Read the model definition and answer for the solid it produces. Units are mm, in the model's axes. A direction names the side the tool comes from. Coordinates: 2 decimals unless noted, no trailing zeros. Write each loop counter-clockwise with the first axis right and the second up, starting at its lowest first coordinate (ties: lowest second). Pieces come first, ordered by that corner, then holes. Notation, with made-up numbers: (-10, 61) - (16, 61) arc R18 cw to (16, 79) - close; hole circle Ø11 at (79.25, -39.5). An arc over 180 degrees is marked (long way). Return JSON: item names as keys, results as strings.
```python
from build123d import *

# Parameters (mm, degrees)
SKETCH1_W           = 69
SKETCH1_H           = 40
BOSS_EXTRUDE1_DEPTH = 5.08
SKETCH2_W           = 23
SKETCH2_H           = 5.08
BOSS_EXTRUDE2_DEPTH = 5.08
CUT_EXTRUDE4_DEPTH  = 5.08


with BuildPart() as part:
    # Sketch1 → Boss-Extrude1 (new body)
    with BuildSketch(Plane(origin=(0, 0, 0), x_dir=(1, 0, 0), z_dir=(0, 1, 0))):
        with Locations((-34.5, 20)):
            Rectangle(SKETCH1_W, SKETCH1_H)
    extrude(amount=BOSS_EXTRUDE1_DEPTH)

    # Sketch2 → Boss-Extrude2 (add)
    with BuildSketch(Plane.XY):
        with Locations((-57.5, 2.54)):
            Rectangle(SKETCH2_W, SKETCH2_H)
        with Locations((-11.5, 2.54)):
            Rectangle(SKETCH2_W, SKETCH2_H)
    extrude(amount=BOSS_EXTRUDE2_DEPTH)

    # Sketch7 → Cut-Extrude4 (cut)
    with BuildSketch(Plane(origin=(0, 5.08, 0), x_dir=(1, 0, 0), z_dir=(0, 1, 0))):
        with BuildLine():
            ThreePointArc((-28.25, 10), (-34.5, 16.25), (-40.75, 10))
            Line((-40.75, 10), (-28.25, 10))
        make_face()
        with BuildLine():
            Line((-28.25, 10), (-40.75, 10))
            ThreePointArc((-40.75, 10), (-34.5, 3.75), (-28.25, 10))
        make_face()
        with BuildLine():
            Line((-40.75, 40), (-40.75, 10))
            ThreePointArc((-40.75, 10), (-34.5, 16.25), (-28.25, 10))
            Line((-28.25, 10), (-28.25, 40))
            Line((-28.25, 40), (-40.75, 40))
        make_face()
    extrude(amount=-CUT_EXTRUDE4_DEPTH, mode=Mode.SUBTRACT)


solid = part.part
```
(1) Which of the six approach directions +Z, -Z, +X, -X, +Y, -Y give full straight-line access (tool end or side, diameter ignored) to faces 4 (the face through (-28.25, 3, -25)), 5 (the face through (-43, 5.08, -18)), 6 (the face through (-46, 3, 3))?
Answer:
{"face 4": "-Z, +Y, -Y", "face 5": "+Z, -Z, +X, -X, +Y", "face 6": "+Z, +Y, -Y"}
(2) Determine the mould class of faces 1 (the face through (-40.75, 3, -25)), 2 (the face through (0, 3, -17)), 3 (the face through (-55, 3, -40)) for opening direction X: +X half, -X half, draft (parallel to the pull), parting line (faces both ways), or undercut.
Answer:
{"face 1": "undercut", "face 2": "+X half", "face 3": "draft"}
(3) A cutting plane is placed at C-C (x = -43.5). Determine the outline of the cut face in (y, z), and give its area (3 significant figures).
Answer:
{"outline": "(0, -40) - (5.08, -40) - (5.08, 0) - (0, 0) - close", "area": "203 mm²"}
(4) A cutting plane is placed at D-D (x = -34.5). Determine the outline of the cut face in (y, z), and give its area (4 significant figures).
Answer:
{"outline": "(0, -3.75) - (5.08, -3.75) - (5.08, 0) - (0, 0) - close", "area": "19.05 mm²"}
(5) Flat-ended cylindrical pins translate along their axes: P1, Ø5, axis at x = -43.5, z = -19.5, coming from the -Y side; P2, Ø2, axis at x = -34.5, y = 2.5, coming from the +Z side. Find the tip coordinate at first contact, or state that the pin passes through.
Answer:
{"P1": "y = 0", "P2": "z = 0"}
(6) A cutting plane is placed at A-A (z = -19.5). Determine the outline of the cut face in (x, y), and give its area (3 significant figures).
Answer:
{"outline": "(-69, 0) - (-40.75, 0) - (-40.75, 5.08) - (-69, 5.08) - close; (-28.25, 0) - (0, 0) - (0, 5.08) - (-28.25, 5.08) - close", "area": "287 mm²"}
(7) Straight lines are drawn through the part: line 1 (X direction, y = 1.55, z = -23); line 2 (X direction, y = 4.45, z = 1); line 3 (Z direction, x = -31.5, y = 1.2). For each, find the intervals that lie inside material, in ascending order. Write a range as from..to.
Answer:
{"line 1": "-69..-40.75, -28.25..0", "line 2": "-69..-46, -23..0", "line 3": "-4.52..0"}
(8) A cutting plane is placed at B-B (y = 3.35). Determine the outline of the cut face in (x, z).
Answer:
{"outline": "(-69, -40) - (-40.75, -40) - (-40.75, -10) arc R6.25 cw to (-28.25, -10) - (-28.25, -40) - (0, -40) - (0, 5.08) - (-23, 5.08) - (-23, 0) - (-46, 0) - (-46, 5.08) - (-69, 5.08) - close"}
